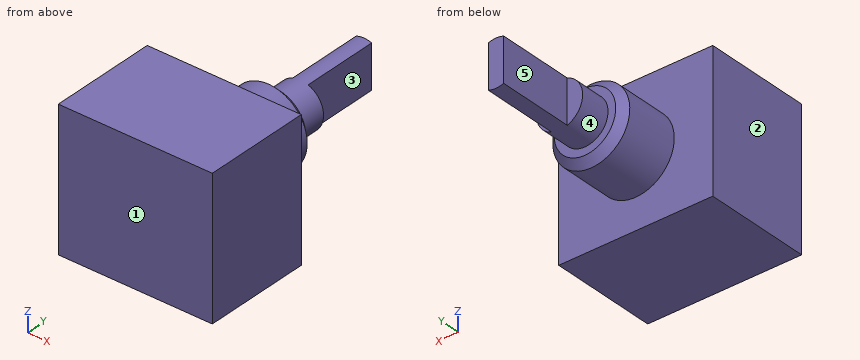
from build123d import *

# Parameters (mm, degrees)
SKETCH_1_W          = 10
SKETCH_1_H          = 9
EXTRUDE_1_DEPTH     = 7
SKETCH_2_R          = 2.5
EXTRUDE_2_DEPTH     = 4
CHAMFER_1_SIZE      = 0.5
SKETCH_3_R          = 1.5
EXTRUDE_3_DEPTH     = 7
CUT_EXTRUDE_START   = -5
CUT_EXTRUDE_1_DEPTH = 5


with BuildPart() as part:
    # 草图1 → 凸台-拉伸1 (new body)
    with BuildSketch(Plane(origin=(0, 0, 0), x_dir=(1, 0, 0), z_dir=(0, 1, 0))):
        Rectangle(SKETCH_1_W, SKETCH_1_H)
    extrude(amount=EXTRUDE_1_DEPTH)

    # 草图2 → 凸台-拉伸2 (add)
    with BuildSketch(Plane(origin=(0, 7, 0), x_dir=(1, 0, 0), z_dir=(0, 1, 0))):
        with Locations(Location((0, 0, 0), (0, 0, 270))):
            Circle(SKETCH_2_R)
    extrude(amount=EXTRUDE_2_DEPTH)

    # 倒角1
    chamfer_1_edges = [part.edges().sort_by_distance(p)[0] for p in [
        (0, 11, -2.5),
    ]]
    chamfer(chamfer_1_edges, length=CHAMFER_1_SIZE)

    # 草图3 → 凸台-拉伸3 (add)
    with BuildSketch(Plane(origin=(0, 11, 0), x_dir=(1, 0, 0), z_dir=(0, 1, 0))):
        with Locations(Location((0, 0, 0), (0, 0, 270))):
            Circle(SKETCH_3_R)
    extrude(amount=EXTRUDE_3_DEPTH)

    # 草图4 → 切除-拉伸1 (cut)
    with BuildSketch(Plane(origin=(0, 18, 0), x_dir=(1, 0, 0), z_dir=(0, 1, 0)).offset(CUT_EXTRUDE_START)):
        with BuildLine():
            Line((-0.5, 1.414213562), (-0.5, -1.414213562))
            ThreePointArc((-0.5, -1.414213562), (-1.5, 0), (-0.5, 1.414213562))
        make_face()
        with BuildLine():
            Line((0.5, 1.414213562), (0.5, -1.414213562))
            ThreePointArc((0.5, -1.414213562), (1.5, 0), (0.5, 1.414213562))
        make_face()
    extrude(amount=CUT_EXTRUDE_1_DEPTH, mode=Mode.SUBTRACT)


solid = part.part
Design review of the part built by this model. Coordinates are the model's own, in mm. Face numbers are marked on the shaded views. A direction names the side the tool comes from. Give positions to 0.01 mm unless a question says otherwise; leave off trailing zeros. Loops run counter-clockwise (first coordinate to the right, second up) from the corner with the lowest first, then second, coordinate; pieces in that order, holes last. Notation, with made-up numbers: M 60.5,16 L 69.5,16 A11 ccw 69.5,21 Z; hole C 32,-28.75 d9. An arc over 180 degrees is marked long. Write item = value, one per line.
Q1. We need section B-B (z = 0). Give the boundary of the cut face in (x, y).
Output values:
outline = M -5,0 L 5,0 L 5,7 L 2.5,7 L 2.5,10.5 L 2,11 L 1.5,11 L 1.5,13 L 0.5,13 L 0.5,18 L -0.5,18 L -0.5,13 L -1.5,13 L -1.5,11 L -2,11 L -2.5,10.5 L -2.5,7 L -5,7 Z
Q2. We need section D-D (y = 12.75). Give the boundary of the cut face in (x, z), plus the area to 3 significant figures.
Output values:
outline = C 0,0 d3
area = 7.07 mm^2
Q3. For the marked faces 1, 2, 3, 4 and 5, list the 3-axis set-ups (+Z, -Z, +X, -X, +Y, -Y) from which the entire face can be reached by the end or side of a thin tool; tool diameter is ignored.
Output values:
face_1 = +Z, -Z, +X, -X, -Y
face_2 = +Z, -Z, -X, +Y, -Y
face_3 = +Z, -Z, +X, +Y
face_4 = +Y
face_5 = +Z, -Z, -X, +Y
Q4. Insertion check: pin 1 (0.8 mm diameter, centred on x = 1, z = -0.5, fed in from +Y); pin 2 (1.4 mm diameter, centred on y = 14.5, z = 0, fed in from +X); pin 3 (3 mm diameter, centred on x = -1, z = 0.5, fed in from +Y); pin 4 (2.5 mm diameter, centred on y = 16, z = 0.5, fed in from -X). Each pin has a flat end and moves straight along its axis. Give the tip position at first contact, or say it passes through.
Output values:
pin_1 = 13
pin_2 = 0.5
pin_3 = 18
pin_4 = -0.5
Q5. We need section A-A (x = 0). Give the boundary of the cut face in (y, z).
Output values:
outline = M 0,-4.5 L 7,-4.5 L 7,-2.5 L 10.5,-2.5 L 11,-2 L 11,-1.5 L 18,-1.5 L 18,1.5 L 11,1.5 L 11,2 L 10.5,2.5 L 7,2.5 L 7,4.5 L 0,4.5 Z
Q6. We need section C-C (y = 9.75). Give the boundary of the cut face in (x, z).
Output values:
outline = C 0,0 d5
Q7. To check wall thickness, follow line 1 (X direction, y = 9.5, z = -1.5); line 2 (Y direction, x = 2, z = 3.5); line 3 (Z direction, x = 0, y = 16.75). State the ranges of each line that lie inside material, in increasing order. Write a range as [from, to].
Output values:
line_1 = [-2, 2]
line_2 = [0, 7]
line_3 = [-1.5, 1.5]
